Can you work these out from the model? Positions are in its coordinate system, mm. A direction names the side the tool comes from. Give positions to 0.01 mm unless a question says otherwise; leave off trailing zeros. Order: outer loops, then holes, each group sorted by start corner. A loop starts at its lowest first (then second) coordinate and runs counter-clockwise, first axis right, second up.
Item 1: I want a section at C-C, the plane z = 3.75. Write out the boundary of the cut face in (x, y), then the cut area to 3 significant figures.
Item 2: I want a section at B-B, the plane z = 7.5. Write out the boundary of the cut face in (x, y), then the cut area to 3 significant figures.
Item 3: If I drill on line 1 along X through (y, z) = (-5.25, 7.5); line 2 along X through (y, z) = (7.5, 11.75); line 3 along Y through (x, z) = (0, 6.25), over which ranges is the centre line in solid material (lowest first)?
Item 4: I want a section at A-A, the plane x = 0. Write out the boundary of the cut face in (y, z).
Item 5: I want a section at D-D, the plane y = 14.5. Write out the boundary of the cut face in (x, z), then the cut area to 3 significant figures.
Item 6: If we mould it in two halves opening along Z, with no side actions, what happens to faces 1 (the flat face through (0, 2, 0)), 2 (the cylindrical face through (-15.017, -5.034, 7.76)), 3 (the cylindrical face through (15.048, -5.046, 7.934)), 4 (the cylindrical face through (11.93, -3.1, 7.6))? For each: +Z half, -Z half, draft (parallel to the pull), parting line (faces both ways), or undercut.
Item 7: I'm going to push flat-ended pins straight in: pin 1 Ø6 at (y, z) = (10.5, 7) entering from -X; pin 2 Ø4 at (x, z) = (7.5, 6) entering from +Y; pin 3 Ø4.5 at (x, z) = (-17, 7.5) entering from +Y. Where does each tip first touch, or does it pass through?
Item 8: Which directions (+Z, -Z, +X, -X, +Y, -Y) give clear straight access to the entire face, cutting with the end or side of a thin tool? Please do faces 5 (the flat face through (0, -2.5, 8)), 6 (the flat face through (-21, -6, 7)).
```python
from build123d import *

# Parameters (mm, degrees)
BOSS_EXTRUDE1_DEPTH     = 15
CUT_EXTRUDE1_DEPTH      = 32.180923655
CUT_EXTRUDE1_DEPTH_BACK = 32.180923655
SKETCH2_R               = 4
CUT_EXTRUDE2_DEPTH      = 32.180923655
CUT_EXTRUDE2_DEPTH_BACK = 32.180923655
CUT_EXTRUDE3_DEPTH      = 36.930488446
CUT_EXTRUDE3_DEPTH_BACK = 36.930488446
SKETCH5_R               = 2
CUT_EXTRUDE4_DEPTH      = 36.930488547
CUT_EXTRUDE4_DEPTH_BACK = 5
SKETCH7_W               = 25
SKETCH7_H               = 15
FILLET1_R               = 2


with BuildPart() as part:
    # Sketch1 → Boss-Extrude1 (new body)
    with BuildSketch(Plane.XY):
        with BuildLine():
            Line((-21, -7.5), (21, -7.5))
            Line((21, -7.5), (21, 7.5))
            Line((21, 7.5), (10, 7.5))
            ThreePointArc((10, 7.5), (0, 17.5), (-10, 7.5))
            Line((-10, 7.5), (-21, 7.5))
            Line((-21, 7.5), (-21, -7.5))
        make_face()
    extrude(amount=BOSS_EXTRUDE1_DEPTH)

    # Sketch2 → Cut-Extrude1 (cut, two sides: drawn at the far end of the back side and taken through both)
    with BuildSketch(Plane.XY.offset(15).offset(-CUT_EXTRUDE1_DEPTH_BACK)):
        with Locations((0, 7.5)):
            Circle(SKETCH2_R)
    extrude(amount=CUT_EXTRUDE1_DEPTH + CUT_EXTRUDE1_DEPTH_BACK, mode=Mode.SUBTRACT)

    # Sketch4 → Cut-Extrude2 (cut, two sides: drawn at the far end of the back side and taken through both)
    with BuildSketch(Plane.XY.offset(15).offset(-CUT_EXTRUDE2_DEPTH_BACK)):
        with BuildLine():
            ThreePointArc((-21, -3.5), (-13.484032178, -0.015967822), (-10, 7.5))
            Line((-10, 7.5), (-21, 7.5))
            Line((-21, 7.5), (-21, -3.5))
        make_face()
        with BuildLine():
            Line((21, 7.5), (10, 7.5))
            ThreePointArc((10, 7.5), (13.484032178, -0.015967822), (21, -3.5))
            Line((21, -3.5), (21, 7.5))
        make_face()
    extrude(amount=CUT_EXTRUDE2_DEPTH + CUT_EXTRUDE2_DEPTH_BACK, mode=Mode.SUBTRACT)

    # Sketch5 → Cut-Extrude3 (cut, two sides: drawn at the far end of the back side and taken through both)
    with BuildSketch(Plane.XZ.offset(7.5).offset(-CUT_EXTRUDE3_DEPTH_BACK)):
        with Locations(Location((-17, 7.5, 0), (0, 0, 270))):
            Circle(SKETCH5_R)
        with Locations(Location((17, 7.5, 0), (0, 0, 270))):
            Circle(SKETCH5_R)
    extrude(amount=CUT_EXTRUDE3_DEPTH + CUT_EXTRUDE3_DEPTH_BACK, mode=Mode.SUBTRACT)

    # Sketch7 → Cut-Extrude4 (cut, two sides: drawn at the far end of the back side and taken through both)
    with BuildSketch(Plane.XZ.offset(7.5).offset(-CUT_EXTRUDE4_DEPTH_BACK)):
        with Locations((0, 7.5)):
            Rectangle(SKETCH7_W, SKETCH7_H)
    extrude(amount=CUT_EXTRUDE4_DEPTH + CUT_EXTRUDE4_DEPTH_BACK, mode=Mode.SUBTRACT)

    # Fillet1
    fillet1_edges = [part.edges().sort_by_distance(p)[0] for p in [
        (-21, -3.5, 7.5),
        (21, -3.5, 7.5),
        (12.5, -2.5, 7.5),
        (-12.5, -2.5, 7.5),
        (12.5, -7.5, 7.5),
        (-12.5, -7.5, 7.5),
    ]]
    fillet(fillet1_edges, radius=FILLET1_R)


solid = part.part
```
Results list:
1. outline: (-21, -7.5) - (-14.5, -7.5) arc R2 ccw to (-12.5, -5.5) - (-12.5, -4.5) arc R2 cw to (-10.5, -2.5) - (10.5, -2.5) arc R2 cw to (12.5, -4.5) - (12.5, -5.5) arc R2 ccw to (14.5, -7.5) - (21, -7.5) - (21, -5.22) arc R2 ccw to (19.43, -3.26) arc R12.04 cw to (10, 7.5) arc R10 ccw to (-10, 7.5) arc R12.04 cw to (-19.43, -3.26) arc R2 ccw to (-21, -5.22) - close; hole circle Ø8 at (0, 7.5)
1. area: 429 mm2
2. outline: (-21, -7.5) - (-19, -7.5) - (-19, -3.16) arc R12.04 cw to (-19.43, -3.26) arc R2 ccw to (-21, -5.22) - close; (-15, -7.5) - (-14.5, -7.5) arc R2 ccw to (-12.5, -5.5) - (-12.5, -4.5) arc R2 cw to (-10.5, -2.5) - (10.5, -2.5) arc R2 cw to (12.5, -4.5) - (12.5, -5.5) arc R2 ccw to (14.5, -7.5) - (15, -7.5) - (15, -1.3) arc R12.04 cw to (10, 7.5) arc R10 ccw to (-10, 7.5) arc R12.04 cw to (-15, -1.3) - close; (19, -7.5) - (21, -7.5) - (21, -5.22) arc R2 ccw to (19.43, -3.26) arc R12.04 cw to (19, -3.16) - close; hole circle Ø8 at (0, 7.5)
2. area: 388 mm2
3. line 1: x = -21 to -19, -15 to -12.5, 12.5 to 15, 19 to 21
3. line 2: x = -10 to -4, 4 to 10
3. line 3: y = -2.5 to 3.5, 11.5 to 17.5
4. outline: (-2.5, 0) - (3.5, 0) - (3.5, 15) - (-2.5, 15) - close; (11.5, 0) - (17.5, 0) - (17.5, 15) - (11.5, 15) - close
5. outline: (-7.14, 0) - (7.14, 0) - (7.14, 15) - (-7.14, 15) - close
5. area: 214 mm2
6. face 1: -Z half
6. face 2: undercut
6. face 3: undercut
6. face 4: draft
7. pin 1: stops at x = -10
7. pin 2: stops at y = 15.85
7. pin 3: stops at y = -1.12
8. face 5: +Z, -Z, -Y
8. face 6: +Z, -Z, -X, +Y, -Y
